Geometry check sheet. Reference: the model listing, model coordinates, mm. Face numbers are marked on the shaded views. A direction names the side the tool comes from. Coordinates: 2 decimals unless noted, no trailing zeros. Order: outer loops, then holes, each group sorted by start corner. A loop starts at its lowest first (then second) coordinate and runs counter-clockwise, first axis right, second up. Notation, with made-up numbers: (-5, 69) - (5, 69) arc R24 cw to (5, 83) - close; hole circle Ø3 at (24, 73). An arc over 180 degrees is marked (long way). Return JSON: item names as keys, results as strings. Group by question number.
Item 1: Draft check along Z on the marked faces 1, 2 and 3. Enter one of: pulls with the +Z half, pulls with the -Z half, needs draft (parallel to the pull), parting line crosses it, or undercut.
Item 2: Tool access check on the marked faces 4, 5, 6, 7 and 8. Record the directions out of +Z, -Z, +X, -X, +Y, -Y that give a thin tool (end or side, any length) a straight path to the whole face; none if there is none.
Item 3: Gauge pin test, flat ends, axial feed: pin 1 (0.6 mm diameter, centred on x = 1.5, y = -1.5, fed in from +Z); pin 2 (1.4 mm diameter, centred on x = 0, z = 0, fed in from +Y); pin 3 (1 mm diameter, centred on x = 0.5, z = 0.5, fed in from +Y). Record the tip position at first contact, or that the pin passes through.
Item 4: Scan lines: probe 1 along X at (y, z) = (3.6, 0); probe 2 along Z at (x, y) = (-1.15, -1.75); probe 3 along Y at (x, z) = (-0.2, -0.9). Record each from-to range of solid material in increasing order.
Item 5: Section check A-A on y = 2.25. Enter the section's corners in (x, z).
from build123d import *

# Parameters (mm, degrees)
SKETCH1_W           = 3.5
SKETCH1_H           = 3.5
BOSS_EXTRUDE1_DEPTH = 1.7
SKETCH2_R           = 1.2
BOSS_EXTRUDE2_DEPTH = 2.69
SKETCH4_R           = 0.25
SKETCH5_R           = 0.381
SKETCH5_W           = 0.5
SKETCH5_H           = 0.5
BOSS_EXTRUDE3_DEPTH = 3
CUT_EXTRUDE1_START  = -0.001
SKETCH6_R           = 1
SKETCH6_R_2         = 0.381
CUT_EXTRUDE1_DEPTH  = 0.001


with BuildPart() as part:
    # Sketch1 → Boss-Extrude1 (new body)
    with BuildSketch(Plane(origin=(0, 0, 0), x_dir=(1, 0, 0), z_dir=(0, 1, 0))):
        Rectangle(SKETCH1_W, SKETCH1_H)
    extrude(amount=BOSS_EXTRUDE1_DEPTH)

    # Sketch2 → Boss-Extrude2 (add)
    with BuildSketch(Plane(origin=(0, 1.7, 0), x_dir=(1, 0, 0), z_dir=(0, 1, 0))):
        with Locations(Location((0, 0, 0), (0, 0, 90))):
            Circle(SKETCH2_R)
    extrude(amount=BOSS_EXTRUDE2_DEPTH)

    # Sketch3 → Cut-Revolve1 (revolve, cut)
    with BuildSketch(Plane(origin=(0, 0, 0), x_dir=(0, 0, -1), z_dir=(1, 0, 0))):
        Polygon((0, 4.39), (0, 4.26), (0.0655, 4.26), (0.1905, 4.043493649), (0.1905, 2.94), (0.8, 2.94), (0.8, 4.39), align=None)
    revolve(axis=Axis((0, 0, 0), (0, 1, 0)), mode=Mode.SUBTRACT)

    # Sketch4 → Revolve1 (revolve)
    with BuildSketch(Plane(origin=(0, 0, 0), x_dir=(0, 0, -1), z_dir=(1, 0, 0)), mode=Mode.PRIVATE) as revolve1_sk:
        with Locations((-1.2, 2.32)):
            Circle(SKETCH4_R)
    revolve(revolve1_sk.sketch.rotate(Axis((0, 0, 0), (0, 1, 0)), 180), axis=Axis((0, 0, 0), (0, 1, 0)))

    # Sketch5 → Boss-Extrude3 (add)
    with BuildSketch(Plane.XZ):
        with Locations(Location((0, 0, 0), (0, 0, 270))):
            Circle(SKETCH5_R)
        with Locations((-1.27, -1.27)):
            Rectangle(SKETCH5_W, SKETCH5_H)
        with Locations((1.27, -1.27)):
            Rectangle(SKETCH5_W, SKETCH5_H)
        with Locations((-1.27, 1.27)):
            Rectangle(SKETCH5_W, SKETCH5_H)
        with Locations((1.27, 1.27)):
            Rectangle(SKETCH5_W, SKETCH5_H)
    extrude(amount=BOSS_EXTRUDE3_DEPTH)

    # Sketch6 → Cut-Extrude1 (cut)
    with BuildSketch(Plane.XZ.offset(CUT_EXTRUDE1_START)):
        with Locations(Location((0, 0, 0), (0, 0, 270))):
            Circle(SKETCH6_R)
        with Locations(Location((0, 0, 0), (0, 0, 270))):
            Circle(SKETCH6_R_2, mode=Mode.SUBTRACT)
    extrude(amount=CUT_EXTRUDE1_DEPTH, mode=Mode.SUBTRACT)


solid = part.part
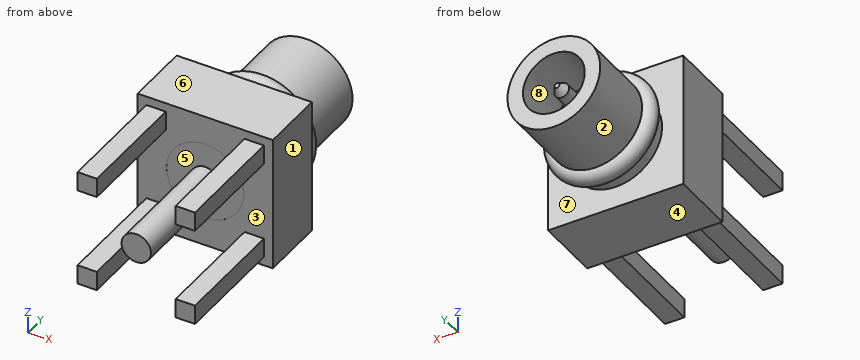
Computed:
{
 "1": {"face 1": "needs draft", "face 2": "parting line crosses it", "face 3": "undercut"},
 "2": {"face 4": "-Z, +X, -X, +Y, -Y", "face 5": "-Y", "face 6": "+Z, +X, -X, +Y, -Y", "face 7": "none", "face 8": "+Y"},
 "3": {"pin 1": "stops at z = 1.52", "pin 2": "stops at y = 4.26", "pin 3": "stops at y = 4.39"},
 "4": {"probe 1": "x = -1.2 to -0.8, -0.19 to 0.19, 0.8 to 1.2", "probe 2": "z = -1.52 to -1.02, 1.02 to 1.52", "probe 3": "y = 0 to 4.39"},
 "5": {"outline": "circle Ø2.88 at (0, 0)"}
}
